Geometry check sheet. Reference: the model listing, model coordinates, mm. A direction names the side the tool comes from. Give positions to 0.01 mm unless a question says otherwise; leave off trailing zeros. Write each loop counter-clockwise with the first axis right and the second up, starting at its lowest first coordinate (ties: lowest second). Pieces come first, ordered by that corner, then holes. Notation, with made-up numbers: (0, 47) -> (46, 47) arc R12 cw to (46, 53) -> close; hole circle Ø2 at (54, 35). An arc over 180 degrees is marked (long way). One line per item, written item: value.
Autodesk Inventor part; units mm, degrees
ref_plane "YZ Plane" through (0, 0, 0) normal (1, 0, 0) x (0, 1, 0)
ref_plane "XZ Plane" through (0, 0, 0) normal (0, 1, 0) x (-1, 0, 0)
ref_plane "XY Plane" through (0, 0, 0) normal (0, 0, 1) x (1, 0, 0)
sketch "Sketch1" plane through (0, 0, 0) normal (0, 1, 0) x (-1, 0, 0)
  line L0 (49, -49) -> (-49, -49)
  line L1 (-49, -49) -> (-49, 49)
  line L2 (-49, 49) -> (49, 49)
  line L3 (49, 49) -> (49, -49)
  circle A0 centre (35, -35) radius 6.5
  circle A1 centre (-35, -35) radius 6.5
  circle A2 centre (-35, 35) radius 6.5
  circle A3 centre (35, 35) radius 6.5
  point P0 (0, 0)
  point P1 (0, -49)
  point P2 (49, 0)
  dimension "d0" = 98
  dimension "d1" = 98
  dimension "d2" = 13
  dimension "d3" = 13
  dimension "d4" = 13
  dimension "d5" = 13
  dimension "d6" = 14
  dimension "d7" = 14
  dimension "d8" = 14
  dimension "d9" = 14
extrude "Extrusion1" add sketch "Sketch1" along normal blind 3
sketch "Sketch2" plane through (0, 3, 0) normal (0, 1, 0) x (1, 0, 0)
  line L0 (-49, -49) -> (49, -49)
  line L1 (-22.5, -49) -> (-22.5, -46)
  line L2 (-22.5, -46) -> (22.5, -46)
  line L3 (22.5, -46) -> (22.5, -49)
  point P0 (0, 0)
  point P1 (0, -46)
  dimension "d12" = 3
  dimension "d13" = 45
extrude "Extrusion2" cut sketch "Sketch2" against normal blind 3
equation "\"d3\" = d2"
equation "\"d4\" = d2"
equation "\"d5\" = d2"
equation "\"d8\" = d6"
equation "\"d9\" = d7"
properties part number "Plate1"
1) Scan lines: probe 1 along Z at (x, y) = (35, 2.15); probe 2 along X at (y, z) = (1.6, -35.5); probe 3 along Z at (x, y) = (-39.5, 1.3). Record each from-to range of solid material in increasing order.
Verdict:
probe 1: -49 to -41.5, -28.5 to 28.5, 41.5 to 49
probe 2: -49 to -41.48, -28.52 to 28.52, 41.48 to 49
probe 3: -49 to -39.69, -30.31 to 30.31, 39.69 to 49
2) Sectioned sample at D-D on x = 10. Record the cut outline in (y, z).
Verdict:
outline: (0, -49) -> (3, -49) -> (3, 46) -> (0, 46) -> close
3) Sectioned sample at C-C on z = -35. Record the cut outline in (x, y).
Verdict:
outline: (-49, 0) -> (-41.5, 0) -> (-41.5, 3) -> (-49, 3) -> close; (-28.5, 0) -> (28.5, 0) -> (28.5, 3) -> (-28.5, 3) -> close; (41.5, 0) -> (49, 0) -> (49, 3) -> (41.5, 3) -> close
4) Sectioned sample at A-A on y = 2.25. Record the cut outline in (x, z), plus the area to 3 significant figures.
Verdict:
outline: (-49, -49) -> (49, -49) -> (49, 49) -> (22.5, 49) -> (22.5, 46) -> (-22.5, 46) -> (-22.5, 49) -> (-49, 49) -> close; hole circle Ø13 at (-35, -35); hole circle Ø13 at (-35, 35); hole circle Ø13 at (35, -35); hole circle Ø13 at (35, 35)
area: 8,940 mm^2
5) Depth check by flat-ended pin: pin 1 Ø1.5 at (x, y) = (20, 2) entering from +Z. Enter the tip coordinate at first touch or a pass-through.
Verdict:
pin 1: z = 46
6) Tool access check on faces 5 (the flat face through (-49, 1, 1)), 6 (the flat face through (0, 2, 46)). Record the directions out of +Z, -Z, +X, -X, +Y, -Y that give a thin tool (end or side, any length) a straight path to the whole face; none if there is none.
Verdict:
face 5: +Z, -Z, -X, +Y, -Y
face 6: +Z, +Y, -Y
7) Mould release check, pull along Z, two halves, no side actions. Record for faces 1 (the flat face through (-1, 1, -49)), 2 (the cylindrical face through (-30.209, 1.479, -39.393)), 3 (the flat face through (49, 1, -1)), 4 (the cylindrical face through (39.791, 1.479, 30.607)): released by +Z, released by -Z, zero draft, split by the parting line, or undercut.
Verdict:
face 1: released by -Z
face 2: undercut
face 3: zero draft
face 4: undercut
8) Sectioned sample at B-B on x = 35. Record the cut outline in (y, z), plus the area to 3 significant figures.
Verdict:
outline: (0, -49) -> (3, -49) -> (3, -41.5) -> (0, -41.5) -> close; (0, -28.5) -> (3, -28.5) -> (3, 28.5) -> (0, 28.5) -> close; (0, 41.5) -> (3, 41.5) -> (3, 49) -> (0, 49) -> close
area: 216 mm^2
